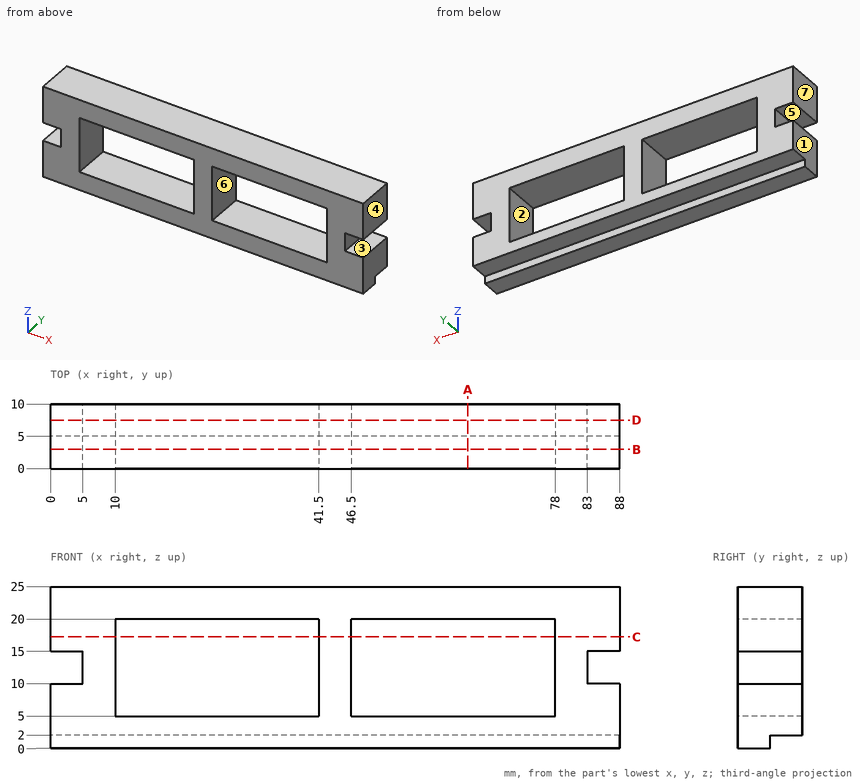
Part print with two shaded views. Sizes in mm from the minimum x, y, z corner. A direction names the side the tool comes from. Give positions to 0.01 mm unless a question says otherwise; leave off trailing zeros. Order: outer loops, then holes, each group sorted by start corner. A loop starts at its lowest first (then second) coordinate and runs counter-clockwise, first axis right, second up. Notation, with made-up numbers: M 29.5,81 L 74.5,81 A27 cw 74.5,111 Z; hole C -35,20.25 d2. An arc over 180 degrees is marked long. Write item = value, one per line.
Q1. Cut at A-A, the plane x = 64.5. List the corners of the cut face in (y, z), then the cut area to 3 significant figures.
Derived:
outline = M 0,0 L 5,0 L 5,2 L 10,2 L 10,5 L 0,5 Z; M 0,20 L 10,20 L 10,25 L 0,25 Z
area = 90.0 mm2
Q2. Tool access for the marked faces 5, 6 and 7: list every direction of +Z, -Z, +X, -X, +Y, -Y with a clear straight run to the whole face (end or side of a thin tool).
Derived:
face_5 = -X, +Y, -Y
face_6 = +Y, -Y
face_7 = +Z, -Z, -X, +Y, -Y
Q3. Cut at D-D, the plane y = 7.5. List the corners of the cut face in (x, z).
Derived:
outline = M 0,2 L 88,2 L 88,10 L 83,10 L 83,15 L 88,15 L 88,25 L 0,25 L 0,15 L 5,15 L 5,10 L 0,10 Z; hole M 10,5 L 41.5,5 L 41.5,20 L 10,20 Z; hole M 46.5,5 L 78,5 L 78,20 L 46.5,20 Z
Q4. Two-plate mould, pull along X, no slides. Class the marked faces 1, 2, 3 and 4: pulls with the +X half, pulls with the -X half, needs draft (parallel to the pull), parting line crosses it, or undercut.
Derived:
face_1 = pulls with the -X half
face_2 = undercut
face_3 = needs draft
face_4 = pulls with the +X half
Q5. Cut at B-B, the plane y = 3. List the corners of the cut face in (x, z).
Derived:
outline = M 0,0 L 88,0 L 88,10 L 83,10 L 83,15 L 88,15 L 88,25 L 0,25 L 0,15 L 5,15 L 5,10 L 0,10 Z; hole M 10,5 L 41.5,5 L 41.5,20 L 10,20 Z; hole M 46.5,5 L 78,5 L 78,20 L 46.5,20 Z
Q6. Cut at C-C, the plane z = 17.25. List the corners of the cut face in (x, y), then the cut area to 3 significant figures.
Derived:
outline = M 0,0 L 10,0 L 10,10 L 0,10 Z; M 41.5,0 L 46.5,0 L 46.5,10 L 41.5,10 Z; M 78,0 L 88,0 L 88,10 L 78,10 Z
area = 250 mm2
Q7. Flat gauge pins, fed straight in: pin 1 (5 mm diameter, centred on x = 58, y = 8, fed in from -Z); pin 2 (1.5 mm diameter, centred on y = 6, z = 12, fed in from +X). Where does each tip first touch, or does it go through?
Derived:
pin_1 = 2
pin_2 = 83
Q8. Drill centre lines: line 1 (X direction, y = 3.75, z = 8); line 2 (Z direction, x = 51.5, y = 5.5); line 3 (Z direction, x = 83.5, y = 0.5). Where is each one in solid material? Low to high. Write a range as [from, to].
Derived:
line_1 = [0, 10], [41.5, 46.5], [78, 88]
line_2 = [2, 5], [20, 25]
line_3 = [0, 10], [15, 25]
